from build123d import *

# Parameters (mm, degrees)
PAD_DEPTH = 5
FILLET_R  = 1


with BuildPart() as part:
    # Sketch → Pad (new body)
    with BuildSketch(Plane.XY):
        with BuildLine():
            ThreePointArc((-9, -17.972479), (0, -20.1), (9, -17.972479))
            Line((9, -21.16601), (9, -17.972479))
            ThreePointArc((6, -22.203603), (7.517922, -21.736625), (9, -21.16601))
            Line((6, -22.203603), (3.888006, -30.939897))
            ThreePointArc((-3.888006, -30.939897), (0, -34), (3.888006, -30.939897))
            Line((-6, -22.203603), (-3.888006, -30.939897))
            ThreePointArc((-9, -21.16601), (-7.517922, -21.736625), (-6, -22.203603))
            Line((-9, -21.16601), (-9, -17.972479))
        make_face()
    extrude(amount=PAD_DEPTH)

    # Fillet
    fillet_edges = [part.edges().sort_by_distance(p)[0] for p in [
        (9, -17.972479, 2.5),
        (9, -21.16601, 2.5),
        (-9, -21.16601, 2.5),
        (-6, -22.203603, 2.5),
        (-9, -17.972479, 2.5),
        (6, -22.203603, 2.5),
    ]]
    fillet(fillet_edges, radius=FILLET_R)


solid = part.part
Part model, mm, in its own coordinate system. Give positions to 0.01 mm unless a question says otherwise; leave off trailing zeros. Order: outer loops, then holes, each group sorted by start corner. A loop starts at its lowest first (then second) coordinate and runs counter-clockwise, first axis right, second up. Notation, with made-up numbers: (33.25, 53.25) -> (50.25, 53.25) arc R9 ccw to (50.25, 63.25) -> close; hole circle Ø9 at (-21.5, 76.5). An arc over 180 degrees is marked (long way). Use one line per item in the form item = value.
(1) Saw through at C-C (x = 2). Write the cut outline in (y, z), then the cut area to 3 significant figures.
Solution:
outline = (-33.46, 0) -> (-20, 0) -> (-20, 5) -> (-33.46, 5) -> close
area = 67.3 mm²
(2) Drill centre lines: line 1 (X direction, y = -30.5, z = 3.75); line 2 (X direction, y = -31.75, z = 3.4); line 3 (Y direction, x = 6.5, z = 0.2). Where is each one in solid material? Low to high. Write a range as from..to.
Solution:
line_1 = -3.99..3.99
line_2 = -3.6..3.6
line_3 = -22.06..-19.02
(3) Saw through at D-D (y = -25). Write the cut outline in (x, z), then the cut area to 3 significant figures.
Solution:
outline = (-5.32, 0) -> (5.32, 0) -> (5.32, 5) -> (-5.32, 5) -> close
area = 53.2 mm²
(4) Saw through at B-B (y = -19.75). Write the cut outline in (x, z), then the cut area to 3 significant figures.
Solution:
outline = (-9, 0) -> (-3.73, 0) -> (-3.73, 5) -> (-9, 5) -> close; (3.73, 0) -> (9, 0) -> (9, 5) -> (3.73, 5) -> close
area = 52.7 mm²
(5) Saw through at A-A (z = 3.15). Write the cut outline in (x, y).
Solution:
outline = (-9, -20.49) arc R1 ccw to (-8.36, -21.43) arc R23 ccw to (-6.55, -22.05) arc R1 cw to (-5.86, -22.77) -> (-3.89, -30.94) arc R4 ccw to (3.89, -30.94) -> (5.86, -22.77) arc R1 cw to (6.55, -22.05) arc R23 ccw to (8.36, -21.43) arc R1 ccw to (9, -20.49) -> (9, -19.52) arc R1 ccw to (7.62, -18.6) arc R20.1 cw to (-7.62, -18.6) arc R1 ccw to (-9, -19.52) -> close
(6) Pull direction X, two halves, no side cores. Call faces 1 (the face through (-9, -20, 2)), 2 (the face through (-0.1, -20.1, 2.5)), 3 (the face through (9, -20, 2)), 4 (the face through (-8.55, -18.69, 2.54)): +X half, -X half, draft (parallel to the pull), parting line (faces both ways), or undercut.
Solution:
face_1 = -X half
face_2 = undercut
face_3 = +X half
face_4 = undercut
(7) Flat gauge pins, fed straight in: P1, Ø1.5, axis at x = -5.5, z = 2, coming from the +Y side; P2, Ø1.5, axis at x = -6, z = 3.5, coming from the +Y side; P3, Ø1.5, axis at x = 4.5, z = 4, coming from the +Y side. Where does each tip first touch, or does it go through?
Solution:
P1 = -19.1
P2 = -18.93
P3 = -19.4
